Work out the finished part from the listing and answer in its coordinate system (mm). A direction names the side the tool comes from. Round coordinates to 2 decimals unless told otherwise and drop trailing zeros. Order: outer loops, then holes, each group sorted by start corner. A loop starts at its lowest first (then second) coordinate and runs counter-clockwise, first axis right, second up. Notation, with made-up numbers: (46, 36) - (104, 36) arc R20 cw to (104, 64) - close; hole circle Ø9 at (-35.75, 1.25). An arc over 180 degrees is marked (long way). Put each result on its own line as item: value.
```python
from build123d import *

# Parameters (mm, degrees)
F1_DEPTH = 3.048


with BuildPart() as f1:
    # F0 (on Top) → F1 (new body)
    with BuildSketch(Plane.XY):
        Polygon((-99.695, 0), (0, 0), (0, 22.86), (-99.695, 22.86), (-99.695, 16.1925), (-99.695, 11.43), (-99.695, 6.6675), align=None)
        Polygon((-104.14, 8.255), (-99.695, 6.6675), (-99.695, 11.43), (-104.14, 11.43), align=None)
        Polygon((-104.14, 11.43), (-99.695, 11.43), (-99.695, 16.1925), (-104.14, 14.605), align=None)
    extrude(amount=-F1_DEPTH)


solid = f1.part
```
1) A cutting plane is placed at B-B on y = 5.5. Write down the section's boundary in (x, z) (3 decimals).
Findings below:
outline: (-99.695, -3.048) - (0, -3.048) - (0, 0) - (-99.695, 0) - close
2) A straight line is drawn through the part: L1, parallel to X at y = 4, z = -2.45 (3 decimals). Find the intervals that lie inside material, in ascending order. Write a range as from..to.
Findings below:
L1: x = -99.695..0
3) A cutting plane is placed at A-A on z = -1.55. Write down the section's boundary in (x, y) (1 decimal).
Findings below:
outline: (-104.1, 8.3) - (-99.7, 6.7) - (-99.7, 0) - (0, 0) - (0, 22.9) - (-99.7, 22.9) - (-99.7, 16.2) - (-104.1, 14.6) - close
4) For faces 1 (the flat face through (-99.695, 20, -2)), 2 (the flat face through (-53, 12, -3.048)), 3 (the flat face through (-99.695, 3, -2)), determine the directions among +Z, -Z, +X, -X, +Y, -Y from which every point of the face is accessible in a straight line to the end or side of a thin tool.
Findings below:
face 1: +Z, -Z, -X, +Y
face 2: -Z, +X, -X, +Y, -Y
face 3: +Z, -Z, -X, -Y
